from build123d import *

# Parameters (mm, degrees)
SKETCH1_R           = 4
SKETCH1_R_2         = 18
BOSS_EXTRUDE1_DEPTH = 8


with BuildPart() as part:
    # Sketch1 → Boss-Extrude1 (new body)
    with BuildSketch(Plane(origin=(0, 0, 0), x_dir=(0, 0, -1), z_dir=(1, 0, 0))):
        with BuildLine():
            ThreePointArc((-38.75, 6.495190528), (-42.5, 0), (-38.75, -6.495190528))
            Line((-38.75, -6.495190528), (-12.5, -21.650635095))
            ThreePointArc((-12.5, -21.650635095), (0, -25), (12.5, -21.650635095))
            Line((12.5, -21.650635095), (38.75, -6.495190528))
            ThreePointArc((38.75, -6.495190528), (42.5, 0), (38.75, 6.495190528))
            Line((38.75, 6.495190528), (12.5, 21.650635095))
            ThreePointArc((12.5, 21.650635095), (0, 25), (-12.5, 21.650635095))
            Line((-12.5, 21.650635095), (-38.75, 6.495190528))
        make_face()
        with Locations((-35, 0)):
            Circle(SKETCH1_R, mode=Mode.SUBTRACT)
        Circle(SKETCH1_R_2, mode=Mode.SUBTRACT)
        with Locations((35, 0)):
            Circle(SKETCH1_R, mode=Mode.SUBTRACT)
    extrude(amount=BOSS_EXTRUDE1_DEPTH)


solid = part.part
Geometry check sheet. Reference: the model listing, model coordinates, mm. Coordinates: 2 decimals unless noted, no trailing zeros. Write each loop counter-clockwise with the first axis right and the second up, starting at its lowest first coordinate (ties: lowest second). Pieces come first, ordered by that corner, then holes. Notation, with made-up numbers: (84.5, -31.5) -> (91.5, -31.5) arc R17 ccw to (91.5, -7.5) -> close; hole circle Ø6 at (4, -13.75). An arc over 180 degrees is marked (long way). One line per question, with ' | ' between items.
1. Cross-section at C-C on y = 0. Record the cut outline in (x, z).
Answers:
outline: (0, -42.5) -> (8, -42.5) -> (8, -39) -> (0, -39) -> close; (0, -31) -> (8, -31) -> (8, -18) -> (0, -18) -> close; (0, 18) -> (8, 18) -> (8, 31) -> (0, 31) -> close; (0, 39) -> (8, 39) -> (8, 42.5) -> (0, 42.5) -> close
2. Cross-section at D-D on y = -9.5. Record the cut outline in (x, z), and give its area (3 significant figures).
Answers:
outline: (0, -33.55) -> (8, -33.55) -> (8, -15.29) -> (0, -15.29) -> close; (0, 15.29) -> (8, 15.29) -> (8, 33.55) -> (0, 33.55) -> close | area: 292 mm²
3. Depth check by flat-ended pin: pin 1 Ø2 at (x, y) = (2, -17.5) entering from +Z; pin 2 Ø6.5 at (y, z) = (0, 35) entering from -X; pin 3 Ø1.5 at (x, y) = (2.5, -11.5) entering from +Z; pin 4 Ø6 at (y, z) = (13, 23.5) entering from -X. Enter the tip coordinate at first touch or a pass-through.
Answers:
pin 1: stops at z = 21.42 | pin 2: passes through | pin 3: stops at z = 31.38 | pin 4: stops at x = 0
4. Cross-section at A-A on z = 0. Record the cut outline in (x, y), and give its area (3 significant figures).
Answers:
outline: (0, -25) -> (8, -25) -> (8, -18) -> (0, -18) -> close; (0, 18) -> (8, 18) -> (8, 25) -> (0, 25) -> close | area: 112 mm²
5. Draft check along Z on faces 1 (the cylindrical face through (4, 25, 0)), 2 (the cylindrical face through (3.9, -2.4, -31.8)), 3 (the flat face through (3.944, 13.967, -25.809)), 4 (the cylindrical face through (3.9, -2.4, 38.2)). Enter one of: +Z half, -Z half, draft (parallel to the pull), parting line (faces both ways), or undercut.
Answers:
face 1: parting line | face 2: undercut | face 3: -Z half | face 4: undercut
6. Thickness scan on probe 1 along Y at (x, z) = (5.5, 0); probe 2 along Z at (x, y) = (5.5, 1); probe 3 along Y at (x, z) = (2.5, -35). Record the ranges inside material, lowest first. Write a range as from..to.
Answers:
probe 1: y = -25..-18, 18..25 | probe 2: z = -42.43..-38.87, -31.13..-17.97, 17.97..31.13, 38.87..42.43 | probe 3: y = -8.66..-4, 4..8.66
7. Cross-section at B-B on x = 4.75. Record the cut outline in (y, z), and give its area (3 significant figures).
Answers:
outline: (-21.65, -12.5) -> (-6.5, -38.75) arc R7.5 ccw to (6.5, -38.75) -> (21.65, -12.5) arc R25 ccw to (21.65, 12.5) -> (6.5, 38.75) arc R7.5 ccw to (-6.5, 38.75) -> (-21.65, 12.5) arc R25 ccw to start; hole circle Ø36 at (0, 0); hole circle Ø8 at (0, -35); hole circle Ø8 at (0, 35) | area: 1,620 mm²
